The listing builds one solid part. Answer for the finished solid, in the listing's coordinates (mm). A direction names the side the tool comes from. Give positions to 0.01 mm unless a question says otherwise; leave off trailing zeros. Loops run counter-clockwise (first coordinate to the right, second up) from the corner with the lowest first, then second, coordinate; pieces in that order, holes last. Notation, with made-up numbers: M 40.5,63 L 64.5,63 A13 ccw 64.5,73 Z; hole C 86,40 d7. An arc over 180 degrees is marked long. Use one line per item in the form item = value. Start each with the question number.
1. Each of these flat-tipped pins is pushed along its axis until it touches: pin 1 Ø2.5 at (y, z) = (3, -74) entering from -X; pin 2 Ø1.5 at (x, y) = (-2, 3.5) entering from -Z; pin 3 Ø1.4 at (y, z) = (2, -68.5) entering from +X; pin 4 Ø6 at (x, z) = (6.5, 21) entering from -Y. Where does it stop, or does it pass through?
2. The part is cut by section D-D (z = -88.5). Write down the section's boundary in (x, y).
3. For faces 4 (the face through (18.1, 2.3, -99.8)), 5 (the face through (0, 0, -8)), 6 (the face through (2.348, 2.382, 4.144)), 7 (the face through (-12.7, 2, -59)), determine the directions among +Z, -Z, +X, -X, +Y, -Y from which every point of the face is accessible in a straight line to the end or side of a thin tool.
4. The mould has two halves that part along Z. Classify faces 1 (the face through (0, 4.699, -8)), 2 (the face through (19.072, 2.317, 69.317)), 3 (the face through (0.33, 2.32, -107.95)): released by +Z, released by -Z, zero draft, split by the parting line, or undercut.
5. The part is cut by section B-B (x = -3). Write down the section's boundary in (y, z).
6. The part is cut by section C-C (x = -19.5). Write down the section's boundary in (y, z), and give its area (3 significant figures).
7. Straight lines are drawn through the part: line 1 (Z direction, x = 0, y = 1.6); line 2 (X direction, y = 0.45, z = -54.5); line 3 (Z direction, x = 4, y = 3.8). For each, find the intervals that lie inside material, in ascending order. Write a range as from..to.
8. The part is cut by section A-A (y = 2.45). Write down the section's boundary in (x, z).
from build123d import *

# Parameters (mm, degrees)
BOSS_EXTRUDE1_DEPTH = 4.699
CUT_EXTRUDE1_REACH  = 112.997


with BuildPart() as part:
    # Sketch2 → Boss-Extrude1 (new body)
    with BuildSketch(Plane(origin=(0, 0, 0), x_dir=(1, 0, 0), z_dir=(0, 1, 0))):
        with BuildLine():
            Line((12.7, 0), (-12.7, 0))
            Line((-12.7, 0), (-12.7, -21.997045256))
            Line((-12.7, -21.997045256), (-12.7, -46.157401043))
            Line((-12.7, -46.157401043), (-12.7, -94.399536545))
            ThreePointArc((-12.7, -94.399536545), (0, -95.25), (12.7, -94.399536545))
            Line((12.7, -94.399536545), (12.7, -46.157401043))
            Line((12.7, -46.157401043), (12.7, -21.997045256))
            Line((12.7, -21.997045256), (12.7, 0))
        make_face()
        with BuildLine():
            Line((-12.7, -94.399536545), (-12.7, -46.157401043))
            Line((-12.7, -46.157401043), (-25.268575407, -91.837147151))
            ThreePointArc((-25.268575407, -91.837147151), (-19.027470653, -93.330155151), (-12.7, -94.399536545))
        make_face()
        with BuildLine():
            Line((25.268575407, -91.837147151), (12.7, -46.157401043))
            Line((12.7, -46.157401043), (12.7, -94.399536545))
            ThreePointArc((12.7, -94.399536545), (19.027470653, -93.330155151), (25.268575407, -91.837147151))
        make_face()
        with BuildLine():
            Line((12.7, 21.997045256), (12.7, 0))
            Line((12.7, 0), (12.7, -21.997045256))
            ThreePointArc((12.7, -21.997045256), (25.4, 0), (12.7, 21.997045256))
        make_face()
        with BuildLine():
            Line((-12.7, -21.997045256), (-12.7, 0))
            Line((-12.7, 0), (-12.7, 21.997045256))
            ThreePointArc((-12.7, 21.997045256), (-25.4, 0), (-12.7, -21.997045256))
        make_face()
        with BuildLine():
            Line((-12.7, 21.997045256), (-12.7, 0))
            Line((-12.7, 0), (12.7, 0))
            Line((12.7, 0), (12.7, 21.997045256))
            Line((12.7, 21.997045256), (12.7, 94.399536545))
            Line((12.7, 94.399536545), (23.631994126, 105.331530672))
            ThreePointArc((23.631994126, 105.331530672), (0, 107.95), (-23.631994126, 105.331530672))
            Line((-23.631994126, 105.331530672), (-12.7, 94.399536545))
            Line((-12.7, 94.399536545), (-12.7, 21.997045256))
        make_face()
    extrude(amount=BOSS_EXTRUDE1_DEPTH)

    # Sketch3 → Cut-Extrude1 (cut, up to next)
    with BuildSketch(Plane(origin=(0, 4.699, 0), x_dir=(1, 0, 0), z_dir=(0, 1, 0)), mode=Mode.PRIVATE) as cut_extrude1_sk1:
        Polygon((-4.7625, 2.749630657), (-4.7625, -2.749630657), (0, -5.499261314), (4.7625, -2.749630657), (4.7625, 2.749630657), (0, 5.499261314), align=None)
    cut_extrude1_tool1 = extrude(cut_extrude1_sk1.sketch, amount=-CUT_EXTRUDE1_REACH, mode=Mode.PRIVATE) & part.part
    add(cut_extrude1_tool1.solids().sort_by_distance((0, 4.699, 0))[0], mode=Mode.SUBTRACT)


solid = part.part
Derived:
q1.pin_1 = -12.7
q1.pin_2 = -107.94
q1.pin_3 = 12.7
q1.pin_4 = 0
q2.outline = M -12.7,0 L 12.7,0 L 12.7,4.7 L -12.7,4.7 Z
q3.face_4 = +X, +Y, -Y
q3.face_5 = +Z, -Z, +X, -X, -Y
q3.face_6 = +Y, -Y
q3.face_7 = -X, +Y, -Y
q4.face_1 = zero draft
q4.face_2 = undercut
q4.face_3 = released by -Z
q5.outline = M 0,-107.91 L 4.7,-107.91 L 4.7,-3.77 L 0,-3.77 Z; M 0,3.77 L 4.7,3.77 L 4.7,95.2 L 0,95.2 Z
q6.outline = M 0,-106.17 L 4.7,-106.17 L 4.7,-101.2 L 0,-101.2 Z; M 0,-16.28 L 4.7,-16.28 L 4.7,16.28 L 0,16.28 Z; M 0,70.87 L 4.7,70.87 L 4.7,93.23 L 0,93.23 Z
q6.area = 281 mm2
q7.line_1 = -107.95..-5.5, 5.5..95.25
q7.line_2 = -12.7..12.7
q7.line_3 = -107.88..-3.19, 3.19..95.17
q8.outline = M -25.27,91.84 L -12.7,46.16 L -12.7,22 A25.4 ccw -12.7,-22 L -12.7,-94.4 L -23.63,-105.33 A107.95 ccw 23.63,-105.33 L 12.7,-94.4 L 12.7,-22 A25.4 ccw 12.7,22 L 12.7,46.16 L 25.27,91.84 A95.25 ccw Z; hole M -4.76,-2.75 L 0,-5.5 L 4.76,-2.75 L 4.76,2.75 L 0,5.5 L -4.76,2.75 Z
